from build123d import *

# Parameters (mm, degrees)
F1_DEPTH = 12
F2_R     = 10


with BuildPart() as f1:
    # F0 (on Front) → F1 (new body)
    with BuildSketch(Plane.XZ):
        with BuildLine():
            Line((-42.918921, -10), (-42.918921, 10))
            ThreePointArc((-42.918921, 10), (-101.203192, 0), (-42.918921, -10))
        make_face()
        Polygon((-86.754676, 8.906493), (-67.538286, 17.542597), (-53.386672, 1.935428), (-63.856883, -16.346437), (-84.479443, -12.038082), align=None, mode=Mode.SUBTRACT)
        with BuildLine():
            Line((40.4763, 10), (-42.918921, 10))
            ThreePointArc((-42.918921, 10), (-41.635235, 5.073059), (-41.203192, 0))
            ThreePointArc((-41.203192, 0), (-41.635235, -5.073059), (-42.918921, -10))
            Line((-42.918921, -10), (40.4763, -10))
            ThreePointArc((40.4763, -10), (37.796808, 0), (40.4763, 10))
        make_face()
        with BuildLine():
            ThreePointArc((-31.200418, -5), (-36.200418, 0), (-31.200418, 5))
            Line((-31.200418, 5), (30.31986, 5))
            ThreePointArc((30.31986, 5), (33.855394, 3.535534), (35.31986, 0))
            ThreePointArc((35.31986, 0), (33.855394, -3.535534), (30.31986, -5))
            Line((30.31986, -5), (-31.200418, -5))
        make_face(mode=Mode.SUBTRACT)
        with BuildLine():
            ThreePointArc((-41.203192, 0), (-41.635235, 5.073059), (-42.918921, 10))
            Line((-42.918921, 10), (-42.918921, -10))
            ThreePointArc((-42.918921, -10), (-41.635235, -5.073059), (-41.203192, 0))
        make_face()
        with BuildLine():
            Line((40.4763, -10), (40.4763, 10))
            ThreePointArc((40.4763, 10), (37.796808, 0), (40.4763, -10))
        make_face()
        with BuildLine():
            ThreePointArc((77.796808, 0), (62.973189, 19.318517), (40.4763, 10))
            Line((40.4763, 10), (40.4763, -10))
            ThreePointArc((40.4763, -10), (62.973189, -19.318517), (77.796808, 0))
        make_face()
        Polygon((45.367177, 8.401368), (61.946016, 14.417447), (72.79079, 0.509104), (62.91439, -14.102803), (45.965665, -9.225116), align=None, mode=Mode.SUBTRACT)
    extrude(amount=F1_DEPTH)

    # F2
    f2_edges = [f1.edges().sort_by_distance(p)[0] for p in [
        (-42.918921, -6, -10),
        (40.4763, -6, -10),
        (40.4763, -6, 10),
        (-42.918921, -6, 10),
    ]]
    fillet(f2_edges, radius=F2_R)


solid = f1.part
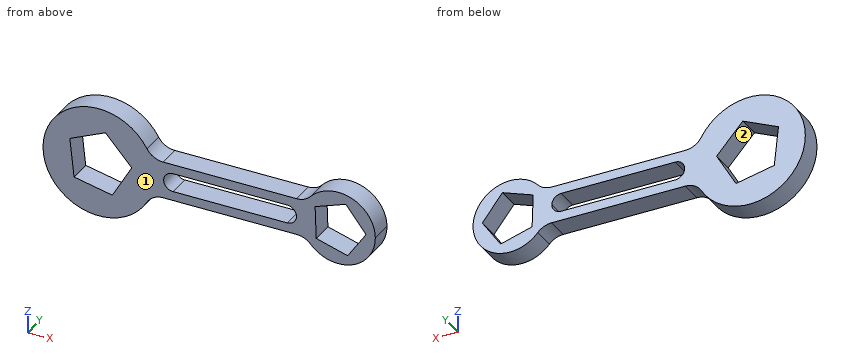
Work out the finished part from the listing and answer in its coordinate system (mm). Face numbers are marked on the shaded views. Coordinates: 2 decimals unless noted, no trailing zeros. Write each loop counter-clockwise with the first axis right and the second up, starting at its lowest first coordinate (ties: lowest second). Pieces come first, ordered by that corner, then holes.
1. The part is cut by section C-C, the plane x = 52. Write down the section's boundary in (y, z).
Results list:
outline: (-12, -19.14) - (0, -19.14) - (0, -10.96) - (-12, -10.96) - close; (-12, 10.81) - (0, 10.81) - (0, 19.14) - (-12, 19.14) - close
2. For a pull along X with two mould halves and no side action, classify the marked faces 1 and 2 as +X half, -X half, draft (parallel to the pull), parting line (faces both ways), or undercut.
Results list:
face 1: draft
face 2: undercut
3. The part is cut by section B-B, the plane y = -8.75. Write down the section's boundary in (x, z).
Results list:
outline: (-45.22, -15) arc R10 cw to (-36.56, -10) - (35.44, -10) arc R10 cw to (42.89, -13.33) arc R20 ccw to (77.8, 0) arc R20 ccw to (42.89, 13.33) arc R10 cw to (35.44, 10) - (-36.56, 10) arc R10 cw to (-45.22, 15) arc R30 ccw (long way) to start; hole (-86.75, 8.91) - (-84.48, -12.04) - (-63.86, -16.35) - (-53.39, 1.94) - (-67.54, 17.54) - close; hole (-31.2, -5) - (30.32, -5) arc R5 ccw to (30.32, 5) - (-31.2, 5) arc R5 ccw to start; hole (45.37, 8.4) - (45.97, -9.23) - (62.91, -14.1) - (72.79, 0.51) - (61.95, 14.42) - close
4. The part is cut by section A-A, the plane x = 27. Write down the section's boundary in (y, z).
Results list:
outline: (-12, -10) - (0, -10) - (0, -5) - (-12, -5) - close; (-12, 5) - (0, 5) - (0, 10) - (-12, 10) - close
5. Flat-ended cylindrical pins translate along their axes: pin 1 (3 mm diameter, centred on y = -6.5, z = 11.5, fed in from -X); pin 2 (6 mm diameter, centred on x = -45.5, y = -8.5, fed in from -Z); pin 3 (6 mm diameter, centred on x = 1.5, y = -7.5, fed in from +Z). Find the tip coordinate at first contact, or state that the pin passes through.
Results list:
pin 1: stops at x = -99.49
pin 2: stops at z = -19.61
pin 3: stops at z = 10
6. Consider line 1 along X through (y, z) = (-10.5, -4); line 2 along Z through (x, y) = (-28, -2.5); line 3 along X through (y, z) = (-3.5, 4). Determine where each line is inside the solid, lowest interval first.
Results list:
line 1: x = -100.94 to -85.35, -56.79 to -34.2, 33.32 to 45.79, 69.74 to 77.39
line 2: z = -10 to -5, 5 to 10
line 3: x = -100.94 to -86.22, -55.26 to -34.2, 33.32 to 45.52, 70.07 to 77.39
7. The part is cut by section D-D, the plane x = -50. Write down the section's boundary in (y, z), and give its area (3 significant figures).
Results list:
outline: (-12, -21.22) - (0, -21.22) - (0, 21.22) - (-12, 21.22) - close
area: 509 mm2
